Could you check a few things on this model? Use its own coordinates, in mm. Face numbers are marked on the shaded views. Round coordinates to 2 decimals unless told otherwise and drop trailing zeros. Loops run counter-clockwise (first coordinate to the right, second up) from the corner with the lowest first, then second, coordinate; pieces in that order, holes last. Notation, with made-up numbers: (49.5, 59.25) - (65.5, 59.25) arc R6 cw to (65.5, 67.25) - close; hole circle Ø1 at (18.5, -4). An arc over 180 degrees is marked (long way). Put each result on its own line as item: value. Start each with the question number.
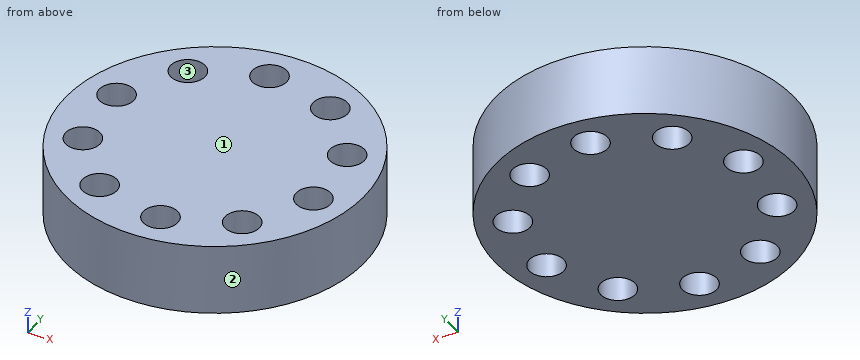
from build123d import *

# Parameters (mm, degrees)
F0_R     = 53.2936931822
F0_R_2   = 6.1448817816
F1_DEPTH = 12.7


with BuildPart() as f1:
    # F0 (on Top) → F1 (new body, symmetric)
    with BuildSketch(Plane.XY):
        Circle(F0_R)
        with Locations((-20.5712730928, -35.6639767333)):
            Circle(F0_R_2, mode=Mode.SUBTRACT)
        with Locations((-37.6052690899, -16.7612723194)):
            Circle(F0_R_2, mode=Mode.SUBTRACT)
        with Locations((4.3202500339, -40.944254209)):
            Circle(F0_R_2, mode=Mode.SUBTRACT)
        with Locations((27.5615844876, -30.5852182209)):
            Circle(F0_R_2, mode=Mode.SUBTRACT)
        with Locations((40.2753304508, -8.5436684258)):
            Circle(F0_R_2, mode=Mode.SUBTRACT)
        with Locations((-40.2753304508, 8.5436684258)):
            Circle(F0_R_2, mode=Mode.SUBTRACT)
        with Locations((-27.5615844876, 30.5852182209)):
            Circle(F0_R_2, mode=Mode.SUBTRACT)
        with Locations((-4.3202500339, 40.944254209)):
            Circle(F0_R_2, mode=Mode.SUBTRACT)
        with Locations((37.6052690899, 16.7612723194)):
            Circle(F0_R_2, mode=Mode.SUBTRACT)
        with Locations((20.5712730928, 35.6639767333)):
            Circle(F0_R_2, mode=Mode.SUBTRACT)
    extrude(amount=F1_DEPTH, both=True)


solid = f1.part
Item 1: Suppose I cut it at B-B, the plane x = 0. List the corners of the cut face in (y, z) for me.
Item 2: I need wall thicknesses on line 1 (X direction, y = 13, z = 9); line 2 (X direction, y = 41, z = -9); line 3 (Y direction, x = 39, z = -1.25). Which ranges of each line are inside material? Lowest first, please. Write a range as from..to.
Item 3: Thinking about a two-plate mould opening in Y: for the marked faces 1, 2 and 3, which applies, released by +Y, released by -Y, zero draft, split by the parting line, or undercut?
Item 4: Will these pins go through, and if not, where does the flat tip stop? P1, Ø10, axis at x = -20.57, y = -35.66, coming from the +Z side; P2, Ø14, axis at x = -4.32, y = 40.94, coming from the +Z side; P3, Ø3, axis at y = -17.5, z = 4.5, coming from the +X side; P4, Ø12, axis at x = -10, z = -7.5, coming from the -Y side.
Item 5: Suppose I cut it at A-A, the plane y = -32. List the corners of the cut face in (x, z) for me.
Item 6: Suppose I cut it at C-C, the plane z = 2.25. Count the separate pieces of the cut face and the enclosed holes in it, then the cut area to 3 significant figures.
Numbers:
1. outline: (-53.29, -12.7) - (-45.31, -12.7) - (-45.31, 12.7) - (-53.29, 12.7) - close; (-36.57, -12.7) - (36.57, -12.7) - (36.57, 12.7) - (-36.57, 12.7) - close; (45.31, -12.7) - (53.29, -12.7) - (53.29, 12.7) - (45.31, 12.7) - close
2. line 1: -51.68..-44.51, -36.04..32.75, 42.46..51.68
2. line 2: -34.05..-10.46, 1.82..17.52, 23.62..34.05
2. line 3: -36.32..-14.55, -2.53..10.78, 22.75..36.32
3. face 1: zero draft
3. face 2: split by the parting line
3. face 3: undercut
4. P1: through
4. P2: z = 12.7
4. P3: x = 50.84
4. P4: y = -53.14
5. outline: (-42.62, -12.7) - (-25.5, -12.7) - (-25.5, 12.7) - (-42.62, 12.7) - close; (-15.64, -12.7) - (21.58, -12.7) - (21.58, 12.7) - (-15.64, 12.7) - close; (33.54, -12.7) - (42.62, -12.7) - (42.62, 12.7) - (33.54, 12.7) - close
6. separate pieces: 1
6. enclosed holes: 10
6. area: 7,740 mm^2
